Can you work these out from the model? Positions are in its coordinate system, mm. A direction names the side the tool comes from. Round coordinates to 2 decimals unless told otherwise and drop trailing zeros. Loops run counter-clockwise (first coordinate to the right, second up) from the corner with the lowest first, then second, coordinate; pieces in that order, holes last. Notation, with made-up numbers: (-2, -18.5) -> (14, -18.5) arc R25 cw to (14, 20.5) -> close; hole circle Ø6 at (9, 15.25). An arc over 180 degrees is marked (long way). Answer as a JSON object with one key per item and string values.
```python
from build123d import *

# Parameters (mm, degrees)
F1_DEPTH = 110
F2_W     = 40
F2_H     = 200
F3_DEPTH = 60
F4_R     = 4.99999
F5_R     = 10


# Not quite as in the source:
# - a fillet or chamfer is up to 0.001 mm smaller than in the source, because OpenCascade refuses the exact size


with BuildPart() as f1:
    # F0 (on Front) → F1 (new body, symmetric)
    with BuildSketch(Plane.XZ):
        Polygon((-30, -60), (30, -60), (30, -50), (30, -45), (25, -45), (25, -50), (-20, -50), (-20, -5), (30, -5), (30, 60), (-30, 60), align=None)
    extrude(amount=F1_DEPTH, both=True)

    # F2 (on face) → F3 (cut)
    with BuildSketch(Plane.XY.offset(60)):
        Rectangle(F2_W, F2_H)
    extrude(amount=-F3_DEPTH, mode=Mode.SUBTRACT)

    # F4 (radius 5 in the source; OpenCascade refuses exactly that, so slightly less here)
    f4_edges = [f1.edges().sort_by_distance(p)[0] for p in [
        (-20, 100, 30),
        (20, 100, 30),
        (-20, -100, 30),
        (20, -100, 30),
        (25, 0, -50),
    ]]
    fillet(f4_edges, radius=F4_R)

    # F5
    f5_edges = [f1.edges().sort_by_distance(p)[0] for p in [
        (30, -110, 27.5),
        (30, 110, 27.5),
    ]]
    fillet(f5_edges, radius=F5_R)


solid = f1.part
```
Q1. We'd pull the mould along Z, two halves only. Please class faces 5 (the flat face through (0, -2, -50)), 6 (the flat face through (-7, 110, 14)), 7 (the flat face through (0, 1, 0)): pulls with the +Z half, pulls with the -Z half, needs draft (parallel to the pull), parting line crosses it, or undercut.
Determined:
{"face 5": "undercut", "face 6": "needs draft", "face 7": "pulls with the +Z half"}
Q2. I want a section at B-B, the plane x = 3.5. Write out the boundary of the cut face in (y, z), then the cut area to 3 significant figures.
Determined:
{"outline": "(-110, -60) -> (110, -60) -> (110, -50) -> (-110, -50) -> close; (-110, -5) -> (110, -5) -> (110, 60) -> (100, 60) -> (100, 0) -> (-100, 0) -> (-100, 60) -> (-110, 60) -> close", "area": "4,500 mm²"}
Q3. I'm going to push flat-ended pins straight in: pin 1 (1 mm diameter, centred on y = 1, z = -43, fed in from +X); pin 2 (20 mm diameter, centred on x = 7.5, y = -44, fed in from +Z). Where does each tip first touch, or does it pass through?
Determined:
{"pin 1": "x = -20", "pin 2": "z = 0"}
Q4. I want a section at A-A, the plane z = 3.5. Write out the boundary of the cut face in (x, y), then the cut area to 3 significant figures.
Determined:
{"outline": "(-30, -110) -> (20, -110) arc R10 ccw to (30, -100) -> (30, 100) arc R10 ccw to (20, 110) -> (-30, 110) -> close; hole (-20, -95) arc R5 ccw to (-15, -100) -> (15, -100) arc R5 ccw to (20, -95) -> (20, 95) arc R5 ccw to (15, 100) -> (-15, 100) arc R5 ccw to (-20, 95) -> close", "area": "5,180 mm²"}
Q5. On a 3-axis mill with a long thin cutter (end or side, diameter ignored), from which of +Z, -Z, +X, -X, +Y, -Y can I reach the whole of each face in a straight line? I mean faces 1 (the cylindrical face through (26.99, 107.15, 27.96)), 2 (the flat face through (28, -2, -45)), 3 (the cylindrical face through (27.15, -106.99, 27.96)), 4 (the cylindrical face through (-18, -99, 30)). Say none if no direction works.
Determined:
{"face 1": "+Z, +X, +Y", "face 2": "+X, +Y, -Y", "face 3": "+Z, +X, -Y", "face 4": "+Z"}
Q6. I want a section at D-D, the plane z = -14.5. Write out the boundary of the cut face in (x, y).
Determined:
{"outline": "(-30, -110) -> (-20, -110) -> (-20, 110) -> (-30, 110) -> close"}
Q7. If I drill on L1, parallel to Z at x = 27.5, y = 25.5; L2, parallel to Y at x = -4, z = 42; L3, parallel to X at y = 36, z = 24, over which ranges is the centre line in solid material (lowest first)? Write a range as [from, to].
Determined:
{"L1": "[-60, -45], [-5, 60]", "L2": "[-110, -100], [100, 110]", "L3": "[-30, -20], [20, 30]"}
